Source: CAD feature listing. Evaluate the final solid. Frame: model axes, mm. A direction names the side the tool comes from. Give positions to 0.01 mm unless a question says otherwise; leave off trailing zeros. Write each loop counter-clockwise with the first axis right and the second up, starting at its lowest first coordinate (ties: lowest second). Pieces come first, ordered by that corner, then holes. Notation, with made-up numbers: M -9,80 L 18,80 A25 cw 18,93 Z; hole C -33,-6.5 d8. An arc over 180 degrees is marked long. Answer as a JSON object with one key per item and string values. Group by question number.
Autodesk Inventor part; units mm, degrees
ref_plane "YZ Plane" through (0, 0, 0) normal (1, 0, 0) x (0, 1, 0)
ref_plane "XZ Plane" through (0, 0, 0) normal (0, 1, 0) x (-1, 0, 0)
ref_plane "XY Plane" through (0, 0, 0) normal (0, 0, 1) x (1, 0, 0)
sketch "草图1" plane through (0, 0, 0) normal (0, 0, 1) x (1, 0, 0)
  circle A0 centre (0, 0) radius 4.5
  dimension "d0" = 9
extrude "拉伸1" add sketch "草图1" along normal blind 8
sketch "草图2" plane through (0, 0, 0) normal (0, 0, -1) x (-1, 0, 0)
  circle A0 centre (0, 0) radius 2
  dimension "d3" = 4
extrude "拉伸2" add sketch "草图2" along normal blind 32
thread "螺纹1"
chamfer "倒角1" distance 0.25 angle 45 1 edges at (2, 0, -32)
sketch "草图3" plane through (0, 0, 8) normal (0, 0, 1) x (1, 0, 0)
  line L0 (1.4434, -2.5) -> (-1.4434, -2.5)
  line L1 (-1.4434, -2.5) -> (-2.8868, 0)
  line L2 (-2.8868, 0) -> (-1.4434, 2.5)
  line L3 (-1.4434, 2.5) -> (1.4434, 2.5)
  line L4 (1.4434, 2.5) -> (2.8868, 0)
  line L5 (2.8868, 0) -> (1.4434, -2.5)
  line L6 (0, 0) -> (0, -0.6524)
  point P0 (0, 2.5)
  dimension "d11" = 0.6524
  dimension "d12" = 5
extrude "拉伸3" cut sketch "草图3" against normal blind 5
properties part number "载板滚柱挡板螺钉"
(1) Access query for faces 4 (the flat face through (0, 0, -32)), 5 (the flat face through (-2.155, -1.267, 5.535)). Directions: +Z, -Z, +X, -X, +Y, -Y. A direction counts if a zero-diameter tool reaches every point of the face in a straight line with its end or side. Return the directions, or none.
(2) Pull-direction query (Y, two-part tool) for faces 1 (the cylindrical face through (0, 2, -16)), 2 (the flat face through (0, 0, 3)), 3 (the flat face through (1, -2, 0)); classes: pulls with the +Y half, pulls with the -Y half, needs draft (parallel to the pull), parting line crosses it, or undercut.
(3) Section A-A, the plane x = 0. Return loops of the section in (y, z).
(4) Contact query for flat-ended pins moving along their axis: pin 1 Ø1 at (x, z) = (-1.5, -27) entering from -Y; pin 2 Ø3 at (y, z) = (-0.5, -9.5) entering from -X; pin 3 Ø1.5 at (x, y) = (-2.5, -0.5) entering from -Z; pin 4 Ø1.5 at (x, y) = (-2, 1) entering from +Z. Output: stop coordinate, or through.
(5) Section B-B, the plane z = 2. Return loops of the section in (x, y), plus the area to 3 significant figures.
(6) Ray query, L1, parallel to Z at x = 1, y = -0.25; L2, parallel to Y at x = -0.25, z = 0.5; L3, parallel to Z at x = -3.25, y = 2. Return the intervals inside material, ascending. Write a range as [from, to].
(7) Section D-D, the plane z = -13. Return loops of the section in (x, y).
(8) Section C-C, the plane y = -3.25. Return loops of the section in (x, z), plus the area to 3 significant figures.
Reported:
{
 "1": {"face 4": "-Z, +X, -X, +Y, -Y", "face 5": "+Z"},
 "2": {"face 1": "parting line crosses it", "face 2": "undercut", "face 3": "needs draft"},
 "3": {"outline": "M -4.5,0 L -2,0 L -2,-31.75 L -1.75,-32 L 1.75,-32 L 2,-31.75 L 2,0 L 4.5,0 L 4.5,8 L 2.5,8 L 2.5,3 L -2.5,3 L -2.5,8 L -4.5,8 Z"},
 "4": {"pin 1": "stops at y = -1.73", "pin 2": "stops at x = -2", "pin 3": "stops at z = -31.95", "pin 4": "stops at z = 8"},
 "5": {"outline": "C 0,0 d9", "area": "63.6 mm2"},
 "6": {"L1": "z = [-32, 3]", "L2": "y = [-4.49, 4.49]", "L3": "z = [0, 8]"},
 "7": {"outline": "C 0,0 d4"},
 "8": {"outline": "M -3.11,0 L 3.11,0 L 3.11,8 L -3.11,8 Z", "area": "49.8 mm2"}
}
